Design review of the part shown in the three views and the two pictorial views. Dimensions are in mm from the part's minimum x, y and z. Give positions to 0.01 mm unless a question says otherwise; leave off trailing zeros. Write each loop counter-clockwise with the first axis right and the second up, starting at its lowest first coordinate (ties: lowest second). Pieces come first, ordered by that corner, then holes. Notation, with made-up numbers: M 69.25,-6 L 95.25,-6 A31 cw 95.25,23 Z; hole C -14,73.25 d10. An arc over 180 degrees is marked long. Use one line per item in the form item = value. Start each with the question number.
Q1. Consider section D-D on y = 53.5. Write out the cut boundary in (x, z).
Q2. Mouldability with a two-part tool opening along Y and no side actions: class the marked faces 1, 2 and 3 as released by +Y, released by -Y, zero draft, split by the parting line, or undercut.
Q3. For probe 1 along Z at (x, y) = (9.75, 7); probe 2 along Y at (x, z) = (9.5, 21.5); probe 3 along X at (y, z) = (55, 38.5), list the stretches that pass through material, from the lowest coordinate up. Write a range as [from, to].
Q4. Consider section A-A on z = 43.18. Give the number of separate pieces and of enclosed holes in the cut face.
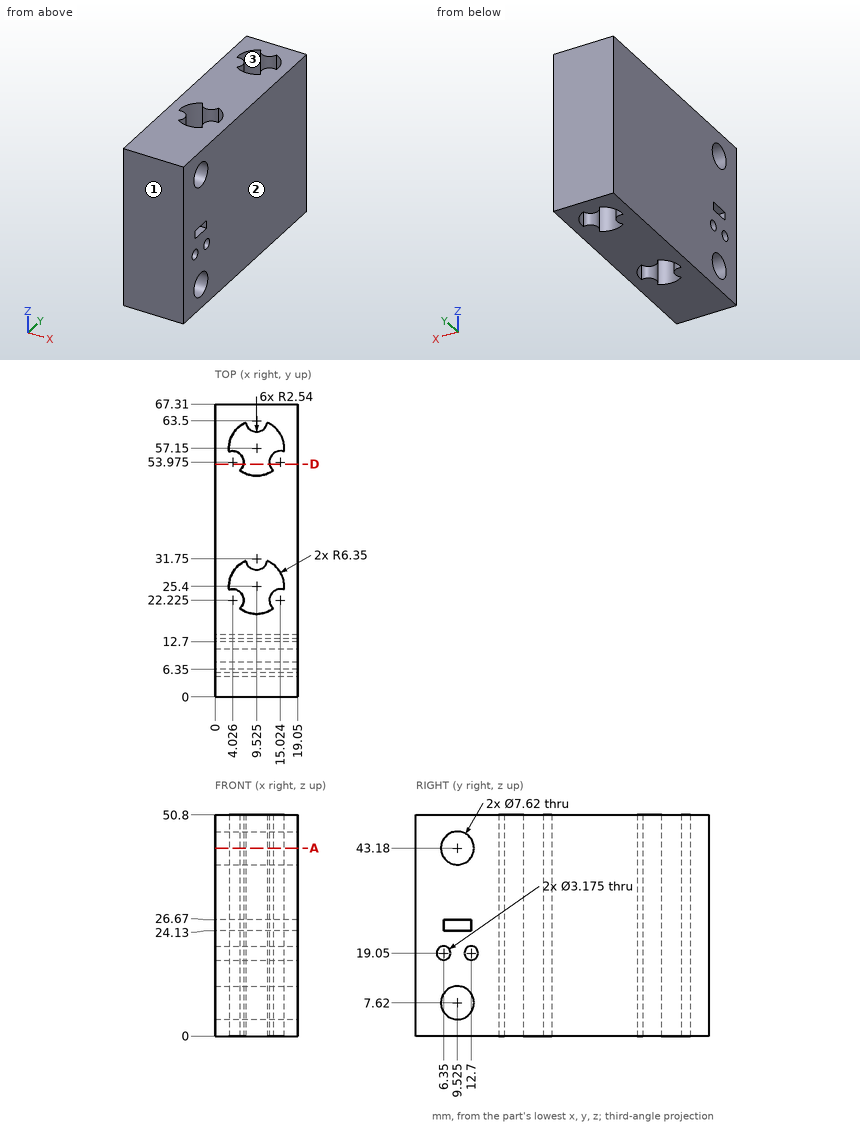
Working result:
q1.outline = M 0,0 L 6.52,0 L 6.52,50.8 L 0,50.8 Z; M 12.53,0 L 19.05,0 L 19.05,50.8 L 12.53,50.8 Z
q2.face_1 = released by -Y
q2.face_2 = zero draft
q2.face_3 = undercut
q3.probe_1 = [0, 4.77], [10.47, 17.6], [20.5, 24.13], [26.67, 40.33], [46.03, 50.8]
q3.probe_2 = [0, 19.05], [29.21, 50.8], [60.96, 67.31]
q3.probe_3 = [0, 6.35], [12.7, 19.05]
q4.separate_pieces = 2
q4.enclosed_holes = 2
